Part print with two shaded views. Sizes in mm from the minimum x, y, z corner. A direction names the side the tool comes from. Give positions to 0.01 mm unless a question says otherwise; leave off trailing zeros. Write each loop counter-clockwise with the first axis right and the second up, starting at its lowest first coordinate (ties: lowest second). Pieces come first, ordered by that corner, then holes.
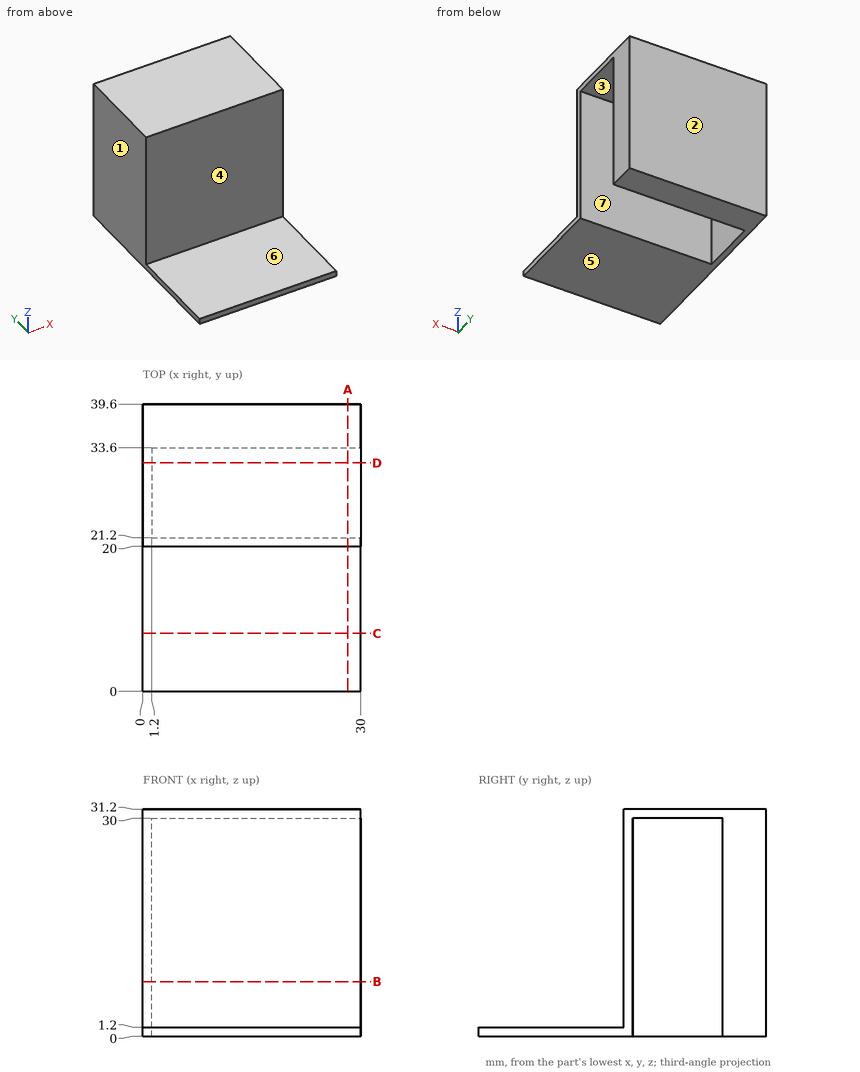
1) Saw through at B-B, the plane z = 7.5. Write the cut outline in (x, y), then the cut area to 3 significant figures.
Answers follow:
outline: (0, 20) - (30, 20) - (30, 21.2) - (1.2, 21.2) - (1.2, 33.6) - (30, 33.6) - (30, 39.6) - (0, 39.6) - close
area: 231 mm2
2) Wall check: L1, parallel to Y at x = 22.75, z = 6; L2, parallel to Z at x = 24, y = 4. Give the ranges that are in metal, low to high.
Answers follow:
L1: y = 20 to 21.2, 33.6 to 39.6
L2: z = 0 to 1.2
3) Saw through at C-C, the plane y = 8. Write the cut outline in (x, z), then the cut area to 3 significant figures.
Answers follow:
outline: (0, 0) - (30, 0) - (30, 1.2) - (0, 1.2) - close
area: 36.0 mm2
4) Saw through at D-D, the plane y = 31.5. Write the cut outline in (x, z).
Answers follow:
outline: (0, 0) - (1.2, 0) - (1.2, 30) - (30, 30) - (30, 31.2) - (0, 31.2) - close
5) 3-axis set-ups, long thin cutter, end or side, ignore diameter. For the marked faces 5, 6 and 7: which of +Z, -Z, +X, -X, +Y, -Y reach the whole face in a straight line?
Answers follow:
face 5: -Z, +X, -X, +Y, -Y
face 6: +Z, +X, -X, -Y
face 7: -Z, +X
6) Pin check, flat tips, straight feed: pin 1 Ø1.5 at (x, z) = (5, 4) entering from -Y; pin 2 Ø5 at (y, z) = (35, 12.5) entering from -X; pin 3 Ø3.5 at (x, y) = (13.5, 26.5) entering from -Z; pin 4 Ø3.5 at (y, z) = (28, 19) entering from +X. Stop position of each tip, or through.
Answers follow:
pin 1: stops at y = 20
pin 2: stops at x = 0
pin 3: stops at z = 30
pin 4: stops at x = 1.2
7) Saw through at A-A, the plane x = 28.25. Write the cut outline in (y, z).
Answers follow:
outline: (0, 0) - (21.2, 0) - (21.2, 30) - (33.6, 30) - (33.6, 0) - (39.6, 0) - (39.6, 31.2) - (20, 31.2) - (20, 1.2) - (0, 1.2) - close
8) Two-plate mould, pull along Y, no slides. Class the marked faces 1, 2, 3 and 4: +Y half, -Y half, draft (parallel to the pull), parting line (faces both ways), or undercut.
Answers follow:
face 1: draft
face 2: +Y half
face 3: undercut
face 4: -Y half
